from build123d import *

# Parameters (mm, degrees)
BOSS_EXTRUDE1_DEPTH                             = 6.35
CBORE_FOR_10_SOCKET_HEAD_CAP_SCREW1_D           = 5.1054
CBORE_FOR_10_SOCKET_HEAD_CAP_SCREW1_CBORE_D     = 9.525
CBORE_FOR_10_SOCKET_HEAD_CAP_SCREW1_CBORE_DEPTH = 4.826
SKETCH5_W                                       = 9.525
SKETCH5_H                                       = 3.175
FILLET1_R                                       = 0.762


with BuildPart() as part:
    # Sketch1 → Boss-Extrude1 (new body)
    with BuildSketch(Plane(origin=(0, 0, 0), x_dir=(1, 0, 0), z_dir=(0, 1, 0))):
        with BuildLine():
            Line((22.225, -38.1), (-22.225, -38.1))
            ThreePointArc((-22.225, -38.1), (-26.715128061, -36.240128061), (-28.575, -31.75))
            Line((-28.575, -31.75), (-28.575, 31.75))
            ThreePointArc((-28.575, 31.75), (-26.715128061, 36.240128061), (-22.225, 38.1))
            Line((-22.225, 38.1), (22.225, 38.1))
            ThreePointArc((22.225, 38.1), (26.715128061, 36.240128061), (28.575, 31.75))
            Line((28.575, 31.75), (28.575, -31.75))
            ThreePointArc((28.575, -31.75), (26.715128061, -36.240128061), (22.225, -38.1))
        make_face()
    extrude(amount=BOSS_EXTRUDE1_DEPTH)

    # CBORE for #10 Socket Head Cap Screw1 (through all)
    with Locations(Plane(origin=(0, 6.35, 0), x_dir=(1, 0, 0), z_dir=(0, 1, 0))):
        with Locations((-22.225, 31.75), (0, 31.75), (22.225, 31.75), (0, -3.175), (22.225, -3.175), (-22.225, -3.175)):
            CounterBoreHole(CBORE_FOR_10_SOCKET_HEAD_CAP_SCREW1_D / 2, CBORE_FOR_10_SOCKET_HEAD_CAP_SCREW1_CBORE_D / 2, CBORE_FOR_10_SOCKET_HEAD_CAP_SCREW1_CBORE_DEPTH)

    # Cut-Sweep1: sweep along a path in Sketch6
    with BuildLine(Plane.XY) as cut_sweep1_path:
        ThreePointArc((22.225, 6.35), (18.744005193, 1.747870067), (13.244743879, 0))
        Line((13.244743879, 0), (-13.244743879, 0))
        ThreePointArc((-13.244743879, 0), (-18.744005193, 1.747870067), (-22.225, 6.35))
    # Sketch5 → Cut-Sweep1 (sweep, cut)
    with BuildSketch(Plane(origin=(0, 0, 0), x_dir=(0, 0, -1), z_dir=(1, 0, 0))):
        with Locations((20.6375, 1.5875)):
            Rectangle(SKETCH5_W, SKETCH5_H)
        with Locations((-23.3625, 1.5875)):
            Rectangle(SKETCH5_W, SKETCH5_H)
    sweep(path=cut_sweep1_path.line, mode=Mode.SUBTRACT)

    # Fillet1
    fillet1_edges = [part.edges().sort_by_distance(p)[0] for p in [
        (18.744005193, 6.35, 23.3625),
        (-18.744005193, 6.35, 23.3625),
        (18.744005193, 6.35, -20.6375),
        (-18.744005193, 6.35, -20.6375),
    ]]
    fillet(fillet1_edges, radius=FILLET1_R)


solid = part.part
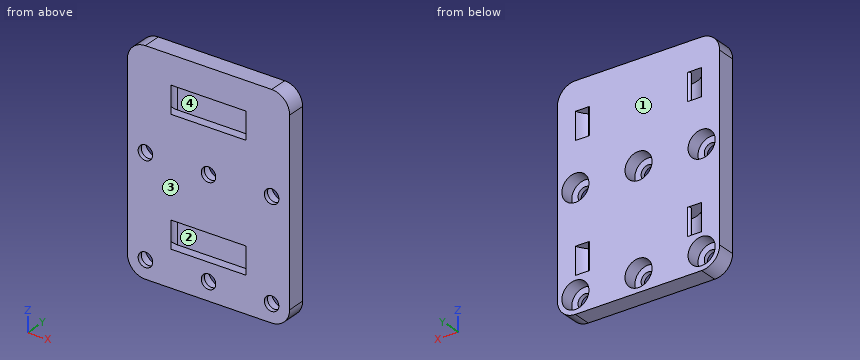
Work out the finished part from the listing and answer in its coordinate system (mm). Face numbers are marked on the shaded views. A direction names the side the tool comes from. Give positions to 0.01 mm unless a question says otherwise; leave off trailing zeros. Write each loop counter-clockwise with the first axis right and the second up, starting at its lowest first coordinate (ties: lowest second). Pieces come first, ordered by that corner, then holes. Notation, with made-up numbers: (82.25, -31.75) - (98.25, -31.75) arc R33 cw to (98.25, 4.25) - close; hole circle Ø2 at (87, -9). An arc over 180 degrees is marked (long way). One line per item, written item: value. Start each with the question number.
1. Find section B-B (z = -19). Write down the section's boundary in (x, y) (3 decimals).
2. For the marked faces 1 and 2, determine the directions among +Z, -Z, +X, -X, +Y, -Y from which every point of the face is accessible in a straight line to the end or side of a thin tool.
3. Find section C-C (x = 23.5). Write down the section's boundary in (y, z), then the cut area to 3 significant figures.
4. Find section A-A (x = 0). State how many separate pieces and enclosed holes the cut face has, then the cut area to 3 significant figures.
5. For a pull along Z with two mould halves and no side action, classify the marked faces 3 and 4 as +Z half, -Z half, draft (parallel to the pull), parting line (faces both ways), or undercut.
6. Consider probe 1 along X at (y, z) = (1.25, -31.75) (3 decimals); probe 2 along Z at (x, y) = (-16.5, 4) (3 decimals); probe 3 along Z at (x, y) = (0, 3.4). Determine where each line is inside the solid, lowest interval first.
7. Given pin 1 (3 mm diameter, centred on x = 23, z = 1.5, fed in from +Y); pin 2 (10.5 mm diameter, centred on x = 22, z = -34, fed in from +Y); pin 3 (4.5 mm diameter, centred on x = -22.225, z = -31.75, fed in from +Y), each flat-ended and moving along its own axis, determine where each tip first touches the part or whether it passes through.
Geometry results:
1. outline: (-28.575, 0) - (-13.245, 0) arc R9.525 cw to (-22.225, 6.35) - (-28.575, 6.35) - close; (-17.751, 5.051) arc R6.35 ccw to (-13.245, 3.175) - (13.245, 3.175) arc R6.35 ccw to (17.751, 5.051) arc R0.762 ccw to (17.21, 6.35) - (-17.21, 6.35) arc R0.762 ccw to start; (13.245, 0) - (28.575, 0) - (28.575, 6.35) - (22.225, 6.35) arc R9.525 cw to start
2. face 1: +Z, -Z, +X, -X, +Y
2. face 2: -Y
3. outline: (0, -37.97) - (6.35, -37.97) - (6.35, -36.34) - (1.52, -36.34) - (1.52, -33.96) - (0, -33.96) - close; (0, -29.54) - (1.52, -29.54) - (1.52, -27.16) - (6.35, -27.16) - (6.35, -1.41) - (1.52, -1.41) - (1.52, 0.96) - (0, 0.96) - close; (0, 5.39) - (1.52, 5.39) - (1.52, 7.76) - (6.35, 7.76) - (6.35, 37.97) - (0, 37.97) - close
3. area: 380 mm2
4. separate pieces: 3
4. enclosed holes: 0
4. area: 316 mm2
5. face 3: draft
5. face 4: undercut
6. probe 1: -28.575 to -24.778, -19.672 to -2.553, 2.553 to 19.672, 24.778 to 28.575
6. probe 2: -38.1 to -25.4, -15.875 to 18.6, 28.125 to 38.1
6. probe 3: -38.1 to -36.51, -26.99 to -1.59, 7.94 to 38.1
7. pin 1: y = 1.52
7. pin 2: y = 6.35
7. pin 3: through
